Geometry: see drawing. Coordinates: mm, zero at the bounding-box minimum. Coordinates: 2 decimals unless noted, no trailing zeros. Loops run counter-clockwise (first coordinate to the right, second up) from the corner with the lowest first, then second, coordinate; pieces in that order, holes last. Notation, with made-up numbers: (69.5, -10.75) - (116.5, -10.75) arc R22 ccw to (116.5, 15.25) - close; hole circle Ø1 at (57.5, -2.75). An arc over 180 degrees is marked (long way). Use one line per item in the form item = value.
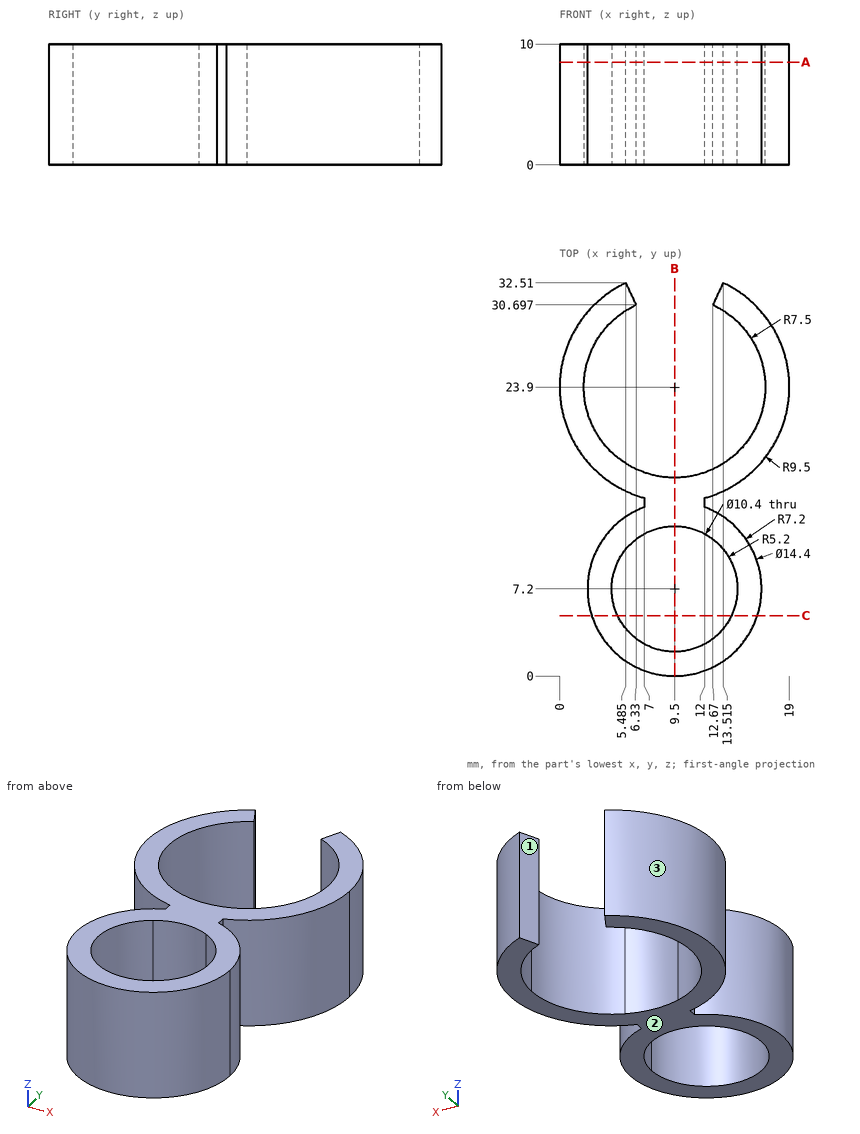
Q1. Pull-direction query (X, two-part tool) for the marked faces 1, 2 and 3; classes: pulls with the +X half, pulls with the -X half, needs draft (parallel to the pull), parting line crosses it, or undercut.
Check values:
face_1 = undercut
face_2 = needs draft
face_3 = pulls with the -X half
Q2. Ray query, line 1 along Y through (x, z) = (6.5, 6.75) (1 decimal); line 2 along Y through (x, z) = (9.75, 8.75) (1 decimal); line 3 along X through (y, z) = (7.2, 3). Return the intervals inside material, ascending. Write a range as [from, to].
Check values:
line_1 = [0.7, 3], [11.4, 13.7], [14.9, 17]
line_2 = [0, 2], [12.4, 16.4]
line_3 = [2.3, 4.3], [14.7, 16.7]
Q3. Cut plane C-C, the plane y = 5. Return loops of the section in (x, z) (1 decimal).
Check values:
outline = (2.6, 0) - (4.8, 0) - (4.8, 10) - (2.6, 10) - close; (14.2, 0) - (16.4, 0) - (16.4, 10) - (14.2, 10) - close
Q4. First-contact query: P1, Ø3, axis at x = 6, z = 8.5, coming from the +Y side; P2, Ø1, axis at y = 20.5, z = 7, coming from the -X side; P3, Ø10, axis at x = 7.5, y = 25.5, coming from the -Z side; P4, Ø1.5, axis at y = 19, z = 3.5, coming from the -X side (1 decimal). Flat tips, straight axial feed; report the tip coordinate or a pass-through.
Check values:
P1 = 32.51
P2 = 0.45
P3 = 0
P4 = 1
Q5. Cut plane B-B, the plane x = 9.5. Return loops of the section in (y, z), then the cut area to 3 significant figures.
Check values:
outline = (0, 0) - (2, 0) - (2, 10) - (0, 10) - close; (12.4, 0) - (16.4, 0) - (16.4, 10) - (12.4, 10) - close
area = 60.0 mm²
Q6. Cut plane A-A, the plane z = 8.5. Return loops of the section in (x, y) (1 decimal).
Check values:
outline = (5.5, 32.5) arc R9.5 ccw to (7, 14.7) - (7, 14) arc R7.2 ccw (long way) to (12, 14) - (12, 14.7) arc R9.5 ccw to (13.5, 32.5) - (12.7, 30.7) arc R7.5 cw (long way) to (6.3, 30.7) - close; hole circle Ø10.4 at (9.5, 7.2)
